```python
from build123d import *

# Parameters (mm, degrees)
F0_W           = 650
F0_H           = 200
F1_DEPTH       = 10
F4_D           = 5
F4_DEPTH       = 20
F4_TIP         = 1.5021515476
F4_ON_F3_D     = 5
F4_ON_F3_DEPTH = 20
F4_ON_F3_TIP   = 1.5021515476
F5_W           = 91
F5_H           = 80
F6_DEPTH       = 25


with BuildPart() as f1:
    # F0 (on Top) → F1 (new body)
    with BuildSketch(Plane.XY):
        Rectangle(F0_W, F0_H)
    extrude(amount=F1_DEPTH)

    # F4
    with Locations(Plane.YZ.offset(325)):
        with Locations((90, 5), (-90, 5)):
            Hole(F4_D / 2, depth=F4_DEPTH)
            with Locations((0, 0, -(F4_DEPTH + F4_TIP / 2))):  # 118° drill point
                Cone(0, F4_D / 2, F4_TIP, mode=Mode.SUBTRACT)

    # F4 on F3
    with Locations(Plane(origin=(-325, 0, 0), x_dir=(0, -1, 0), z_dir=(-1, 0, 0))):
        with Locations((90, 5), (-90, 5)):
            Hole(F4_ON_F3_D / 2, depth=F4_ON_F3_DEPTH)
            with Locations((0, 0, -(F4_ON_F3_DEPTH + F4_ON_F3_TIP / 2))):  # 118° drill point
                Cone(0, F4_ON_F3_D / 2, F4_ON_F3_TIP, mode=Mode.SUBTRACT)

    # F5 (on face) → F6 (cut)
    with BuildSketch(Plane.XY.offset(10)):
        with BuildLine():
            ThreePointArc((-144.4550033747, 33.3169048253), (-167.7112094275, 41.7814723445), (-176.1757760637, 18.5252659703))
            ThreePointArc((-176.1757760637, 18.5252659703), (-152.9195705725, 10.0606996555), (-144.4550033747, 33.3169048253))
        make_face()
        with BuildLine():
            ThreePointArc((-99.1396139363, 54.4478180297), (-122.3958194275, 62.9123843445), (-130.8603866253, 39.6561791747))
            ThreePointArc((-130.8603866253, 39.6561791747), (-107.6041805725, 31.1916116555), (-99.1396139363, 54.4478180297))
        make_face()
        with BuildLine():
            ThreePointArc((-60.6337345533, 31.0267332083), (-83.889940619, 39.4913002552), (-92.3545070637, 16.2350939703))
            ThreePointArc((-92.3545070637, 16.2350939703), (-69.098301381, 7.7705277448), (-60.6337345533, 31.0267332083))
        make_face()
        with BuildLine():
            ThreePointArc((-105.9491247577, 9.8958196467), (-129.2053308382, 18.360386153), (-137.6698970637, -4.8958200297))
            ThreePointArc((-137.6698970637, -4.8958200297), (-114.4136911618, -13.360386153), (-105.9491247577, 9.8958196467))
        make_face()
        with BuildLine():
            ThreePointArc((-53.8242245533, 75.5787312083), (-77.080430619, 84.0432982552), (-85.5449970637, 60.7870919703))
            ThreePointArc((-85.5449970637, 60.7870919703), (-62.288791381, 52.3225257448), (-53.8242245533, 75.5787312083))
        make_face()
        with Locations((-254.5, -30)):
            Rectangle(F5_W, F5_H)
        with BuildLine():
            ThreePointArc((189.369221, 24.921086), (188.954401169, 28.7087790435), (187.7296074467, 32.3169052083))
            ThreePointArc((187.7296074467, 32.3169052083), (168.3260134713, 42.0586377624), (154.3763653155, 25.421086))
            ThreePointArc((154.3763653155, 25.421086), (154.7316693294, 21.3778780275), (156.0088349363, 17.5252659703))
            ThreePointArc((156.0088349363, 17.5252659703), (175.6569144859, 7.835905929), (189.369221, 24.921086))
        make_face()
        with BuildLine():
            ThreePointArc((233.0449962423, 53.4478176467), (209.7887905725, 61.9123843445), (201.3242235533, 38.6561787917))
            ThreePointArc((201.3242235533, 38.6561787917), (224.5804294275, 30.1916116555), (233.0449962423, 53.4478176467))
        make_face()
        with BuildLine():
            ThreePointArc((271.5508764467, 30.0267332083), (248.2946705725, 38.4913003445), (239.8301037577, 15.2350943533))
            ThreePointArc((239.8301037577, 15.2350943533), (263.0863094275, 6.7705276555), (271.5508764467, 30.0267332083))
        make_face()
        with BuildLine():
            ThreePointArc((226.2354870637, 8.8958200297), (202.9792811618, 17.360386153), (194.5147147577, -5.8958196467))
            ThreePointArc((194.5147147577, -5.8958196467), (217.7709208382, -14.360386153), (226.2354870637, 8.8958200297))
        make_face()
        with BuildLine():
            ThreePointArc((278.3603856253, 74.5787308253), (255.1041795725, 83.0432983445), (246.6396129363, 59.7870919703))
            ThreePointArc((246.6396129363, 59.7870919703), (269.8958184275, 51.3225256555), (278.3603856253, 74.5787308253))
        make_face()
        Polygon((32.18461, -70), (32.18461, -71), (123.18461, -71), (123.18461, -70), (123.18461, 9), (32.18461, 9), align=None)
        with BuildLine():
            ThreePointArc((5, 68.182912), (-12.5, 85.682912), (-30, 68.182912))
            ThreePointArc((-30, 68.182912), (-12.5, 50.682912), (5, 68.182912))
        make_face()
        with BuildLine():
            ThreePointArc((56.428404, 68.182912), (38.928404, 85.682912), (21.428404, 68.182912))
            ThreePointArc((21.428404, 68.182912), (38.928404, 50.682912), (56.428404, 68.182912))
        make_face()
    extrude(amount=-F6_DEPTH, mode=Mode.SUBTRACT)


solid = f1.part
```
For this review, take the finished solid that the model builds, in its own axes (mm). Give positions to 0.01 mm unless a question says otherwise; leave off trailing zeros. Write each loop counter-clockwise with the first axis right and the second up, starting at its lowest first coordinate (ties: lowest second). Pieces come first, ordered by that corner, then holes. Notation, with made-up numbers: M -37,12 L 22,12 A19 cw 22,16 Z; hole C -14,20 d2. An arc over 180 degrees is marked long. One line per item, written item: value.
1) Take a section at B-B, the plane x = -12.5. Write out the cut boundary in (y, z), then the cut area to 3 significant figures.
Results are:
outline: M -100,0 L 50.68,0 L 50.68,10 L -100,10 Z; M 85.68,0 L 100,0 L 100,10 L 85.68,10 Z
area: 1,650 mm²
2) For line 1 (Y direction, x = -320.25, z = 5); line 2 (X direction, y = -53.5, z = 0.5); line 3 (Y direction, x = 217.5, z = 6.25), list the stretches that pass through material, from the lowest coordinate up. Write a range as from..to.
Results are:
line 1: y = -100..-92.5, -87.5..87.5, 92.5..100
line 2: x = -325..-300, -209..32.18, 123.18..325
line 3: y = -100..-14.48, 17.48..28.55, 63.55..100
3) The part is to be moulded in two halves that separate along Y. For faces 1 (the flat face through (-5, 1, 10)), 2 (the cylindrical face through (227.063, -3.768, 5.07)), say which applies: +Y half, -Y half, draft (parallel to the pull), parting line (faces both ways), or undercut.
Results are:
face 1: draft
face 2: undercut
4) Take a section at A-A, the plane y = -49.5. Write out the cut boundary in (x, z), then the cut area to 3 significant figures.
Results are:
outline: M -325,0 L -300,0 L -300,10 L -325,10 Z; M -209,0 L 32.18,0 L 32.18,10 L -209,10 Z; M 123.18,0 L 325,0 L 325,10 L 123.18,10 Z
area: 4,680 mm²
5) For P1, Ø21, axis at x = -115, y = 47.05, coming from the +Z side; P2, Ø3, axis at y = 90, z = 5, coming from the +X side; P3, Ø8, axis at x = -17.5, y = -72.5, coming from the -Z side; P4, Ø4, axis at y = -90, z = 5, coming from the +X side, all flat-tipped, find the tip position at first contact; note any pin that passes through.
Results are:
P1: passes through
P2: stops at x = 304.4
P3: stops at z = 0
P4: stops at x = 304.7
6) Take a section at C-C, the plane x = -115. Write out the cut boundary in (y, z).
Results are:
outline: M -100,0 L -13.62,0 L -13.62,10 L -100,10 Z; M 18.62,0 L 29.55,0 L 29.55,10 L 18.62,10 Z; M 64.55,0 L 100,0 L 100,10 L 64.55,10 Z
